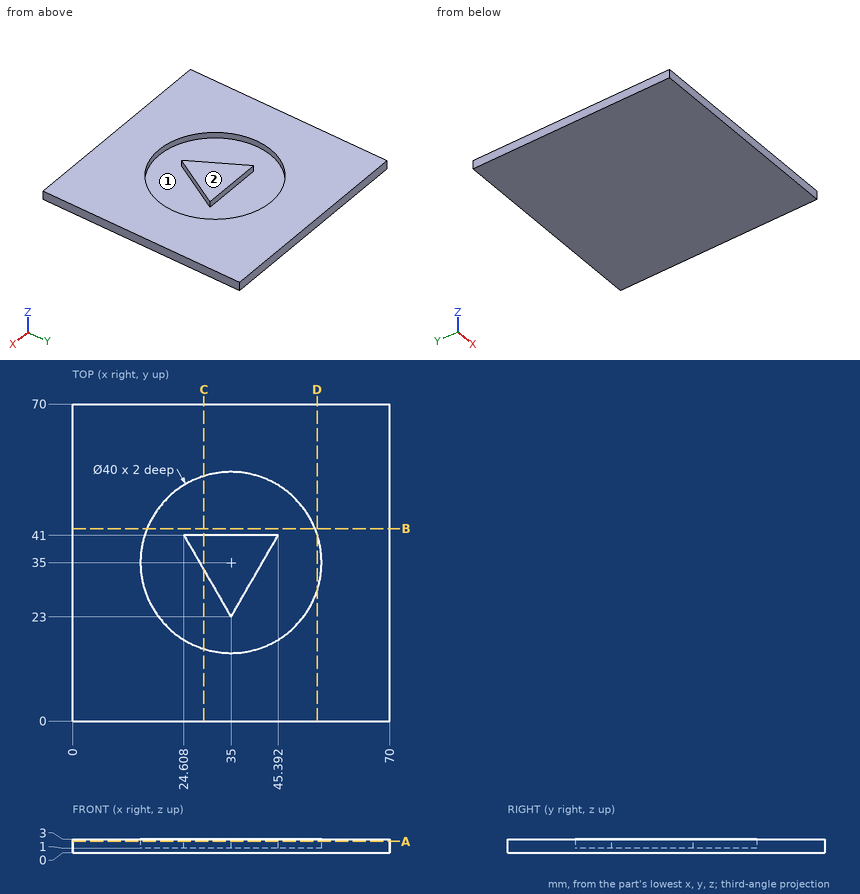
Here's the drawing with two shaded views (mm, measured from the low corner). I have some questions. Give positions to 0.01 mm unless a question says otherwise; leave off trailing zeros. Write each loop counter-clockwise with the first axis right and the second up, starting at its lowest first coordinate (ties: lowest second). Pieces come first, ordered by that corner, then holes. Notation, with made-up numbers: (-13.75, -4.75) -> (6.25, -4.75) arc R17 cw to (6.25, 18.25) -> close; hole circle Ø3 at (50, 11). An arc over 180 degrees is marked (long way). Use one line per item in the form item = value. Start each with the question number.
1. Imagine slicing it at C-C on x = 29. List the corners of the cut face in (y, z) for me, plus the area to 3 significant figures.
2. Imagine slicing it at B-B on y = 42.5. List the corners of the cut face in (x, z) for me, plus the area to 3 significant figures.
3. If I drill on L1, parallel to Y at x = 38.5, z = 2.2; L2, parallel to X at y = 30, z = 1.45 (1 decimal); L3, parallel to Y at x = 31, z = 1.05 (1 decimal), over which ranges is the centre line in solid material (lowest first)?
4. Imagine slicing it at A-A on z = 2.45. List the corners of the cut face in (x, y) for me.
5. Thinking about a two-plate mould opening in X: for the marked faces 1 and 2, which applies, +X half, -X half, draft (parallel to the pull), parting line (faces both ways), or undercut?
6. Imagine slicing it at D-D on x = 54. List the corners of the cut face in (y, z) for me (1 decimal).
Entries:
q1.outline = (0, 0) -> (70, 0) -> (70, 3) -> (54.08, 3) -> (54.08, 1) -> (41, 1) -> (41, 3) -> (33.39, 3) -> (33.39, 1) -> (15.92, 1) -> (15.92, 3) -> (0, 3) -> close
q1.area = 149 mm²
q2.outline = (0, 0) -> (70, 0) -> (70, 3) -> (53.54, 3) -> (53.54, 1) -> (16.46, 1) -> (16.46, 3) -> (0, 3) -> close
q2.area = 136 mm²
q3.L1 = 0 to 15.31, 29.06 to 41, 54.69 to 70
q3.L2 = 0 to 15.6, 31 to 39, 54.4 to 70
q3.L3 = 0 to 15.4, 29.9 to 41, 54.6 to 70
q4.outline = (0, 0) -> (70, 0) -> (70, 70) -> (0, 70) -> close; (24.61, 41) -> (35, 23) -> (45.39, 41) -> close; hole circle Ø40 at (35, 35)
q5.face_1 = undercut
q5.face_2 = draft
q6.outline = (0, 0) -> (70, 0) -> (70, 3) -> (41.2, 3) -> (41.2, 1) -> (28.8, 1) -> (28.8, 3) -> (0, 3) -> close
